```python
from build123d import *

# Parameters (mm, degrees)
F0_W     = 67.056
F0_H     = 138.176
F1_DEPTH = 7.112
F2_R     = 5.08
F3_R     = 4.112792
F4_DEPTH = 0.508
F5_W     = 60.855792
F5_H     = 107.066445
F6_DEPTH = 0.762


with BuildPart() as f1:
    # F0 (on Top) → F1 (new body)
    with BuildSketch(Plane.XY):
        with Locations((5.221646, 24.647108)):
            Rectangle(F0_W, F0_H)
    extrude(amount=F1_DEPTH)

    # F2
    f2_edges = [f1.edges().sort_by_distance(p)[0] for p in [
        (38.749646, 24.647108, 7.112),
        (5.221646, -44.440892, 7.112),
        (-28.306354, 24.647108, 7.112),
        (5.221646, 93.735108, 7.112),
    ]]
    fillet(f2_edges, radius=F2_R)

    # F3 (on face) → F4 (join)
    with BuildSketch(Plane.XY.offset(7.112)):
        with Locations((-17.820586, 83.663628)):
            Circle(F3_R)
    extrude(amount=F4_DEPTH)

    # F5 (on face) → F6 (cut)
    with BuildSketch(Plane(origin=(0, 0, 0), x_dir=(1, 0, 0), z_dir=(0, 0, -1))):
        with Locations((6.081841, -26.345763)):
            Rectangle(F5_W, F5_H)
    extrude(amount=-F6_DEPTH, mode=Mode.SUBTRACT)


solid = f1.part
```
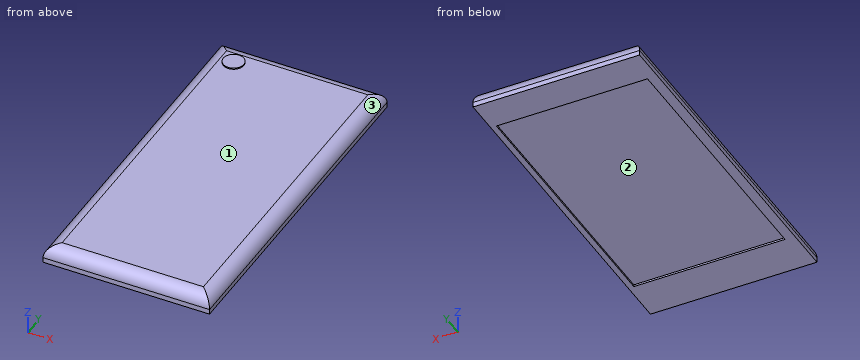
Design review of the part built by this model. Coordinates are the model's own, in mm. Face numbers are marked on the shaded views. Give positions to 0.01 mm unless a question says otherwise; leave off trailing zeros. Write each loop counter-clockwise with the first axis right and the second up, starting at its lowest first coordinate (ties: lowest second). Pieces come first, ordered by that corner, then holes. Notation, with made-up numbers: (-32.5, 78) -> (-21.5, 78) arc R12 ccw to (-21.5, 91) -> close; hole circle Ø11 at (46.5, -17.5). An arc over 180 degrees is marked (long way). Answer in a Markdown table with one row per item.
(1) Consider section C-C (z = 4.75). State the section outline as (x, y) points.
Results:
| item | result |
|---|---|
| outline | (-27.52, -43.65) -> (37.96, -43.65) -> (37.96, 92.95) -> (-27.52, 92.95) -> close |
(2) Consider section B-B (x = 21). State the section outline as (y, z) points, then the cut area to 3 significant figures.
Results:
| item | result |
|---|---|
| outline | (-44.44, 0) -> (-27.19, 0) -> (-27.19, 0.76) -> (79.88, 0.76) -> (79.88, 0) -> (93.74, 0) -> (93.74, 2.03) arc R5.08 ccw to (88.66, 7.11) -> (-39.36, 7.11) arc R5.08 ccw to (-44.44, 2.03) -> close |
| area | 890 mm2 |
(3) Consider section D-D (y = -33.5). State the section outline as (x, z) points, then the cut area to 3 significant figures.
Results:
| item | result |
|---|---|
| outline | (-28.31, 0) -> (38.75, 0) -> (38.75, 2.03) arc R5.08 ccw to (33.67, 7.11) -> (-23.23, 7.11) arc R5.08 ccw to (-28.31, 2.03) -> close |
| area | 466 mm2 |
(4) Clearance check with flat-ended pins moving along their axes: pin 1 (1.5 mm diameter, centred on y = 58.5, z = 6, fed in from +X); pin 2 (17 mm diameter, centred on x = -0.5, y = 26.5, fed in from +Z); pin 3 (1 mm diameter, centred on x = -1.5, z = 6, fed in from +Y). State where each tip first meets the part, or that it passes through.
Results:
| item | result |
|---|---|
| pin 1 | x = 37.6 |
| pin 2 | z = 7.11 |
| pin 3 | y = 92.37 |
(5) To check wall thickness, follow probe 1 along X at (y, z) = (75, 0.5); probe 2 along Z at (x, y) = (28, 55.5); probe 3 along Z at (x, y) = (8.5, -38). State the ranges of each line that lie inside material, in increasing order.
Results:
| item | result |
|---|---|
| probe 1 | -28.31 to -24.35, 36.51 to 38.75 |
| probe 2 | 0.76 to 7.11 |
| probe 3 | 0 to 7.11 |
(6) Mouldability with a two-part tool opening along X and no side actions: class the marked faces 1, 2 and 3 as +X half, -X half, draft (parallel to the pull), parting line (faces both ways), or undercut.
Results:
| item | result |
|---|---|
| face 1 | draft |
| face 2 | undercut |
| face 3 | +X half |
(7) Consider section A-A (y = 41). State the section outline as (x, z) points.
Results:
| item | result |
|---|---|
| outline | (-28.31, 0) -> (-24.35, 0) -> (-24.35, 0.76) -> (36.51, 0.76) -> (36.51, 0) -> (38.75, 0) -> (38.75, 2.03) arc R5.08 ccw to (33.67, 7.11) -> (-23.23, 7.11) arc R5.08 ccw to (-28.31, 2.03) -> close |
